The figure shows three views and two pictorial views of one solid part (mm, origin at its lowest corner). Answer the questions. A direction names the side the tool comes from. Coordinates: 2 decimals unless noted, no trailing zeros. Order: outer loops, then holes, each group sorted by start corner. A loop starts at its lowest first (then second) coordinate and runs counter-clockwise, first axis right, second up.
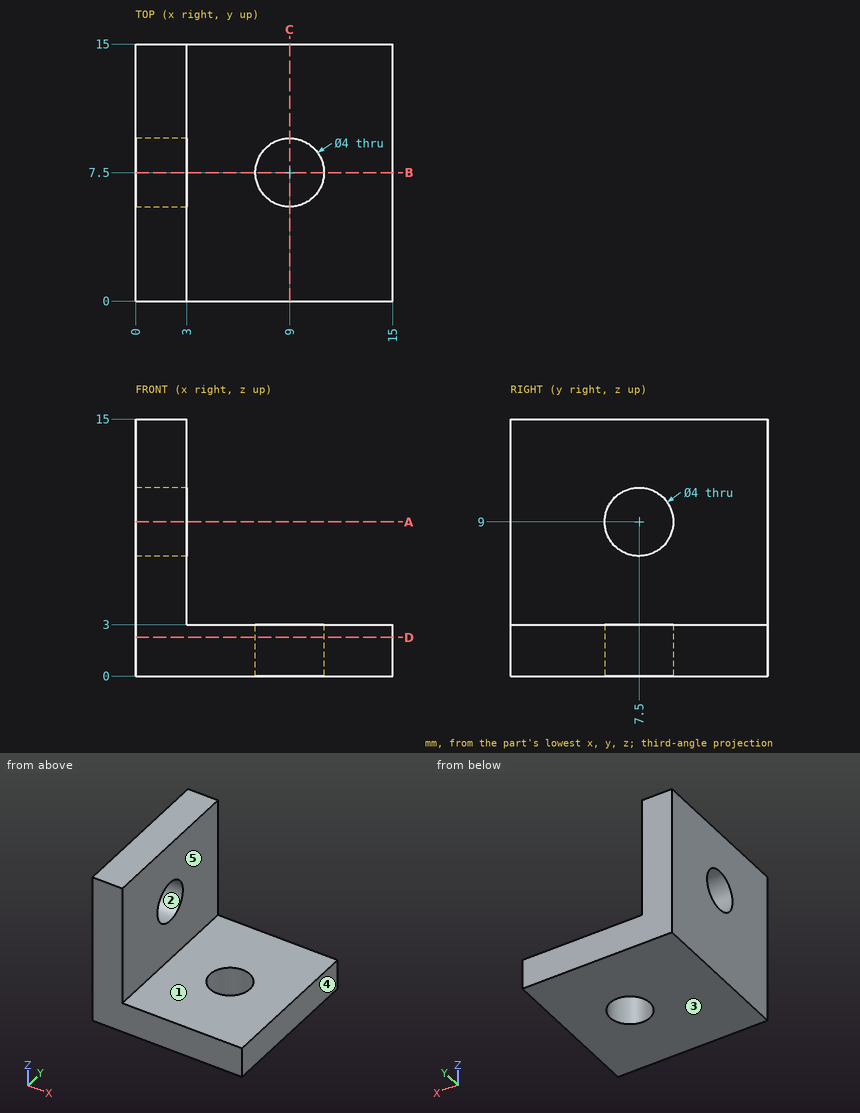
Q1. This flat-tipped pin is pushed along its axis until it touches: P1, Ø1, axis at x = 9.5, y = 7, coming from the +Z side. Where does it stop, or does it pass through?
Q2. The part is cut by section D-D, the plane z = 2.25. Determine the outline of the cut face in (x, y).
Q3. The part is cut by section A-A, the plane z = 9. Determine the outline of the cut face in (x, y), then the cut area to 3 significant figures.
Q4. Determine the mould class of the marked faces 1, 2 and 3 for opening direction Z: +Z half, -Z half, draft (parallel to the pull), parting line (faces both ways), or undercut.
Q5. Straight lines are drawn through the part: L1, parallel to Z at x = 0.75, y = 7.5; L2, parallel to Y at x = 9, z = 0.95; L3, parallel to Z at x = 6.5, y = 6.5. For each, find the intervals that lie inside material, in ascending order.
Q6. Which of the six approach directions +Z, -Z, +X, -X, +Y, -Y give full straight-line access (tool end or side, diameter ignored) to the marked faces 4 and 5?
Q7. The part is cut by section C-C, the plane x = 9. Determine the outline of the cut face in (y, z).
Q8. The part is cut by section B-B, the plane y = 7.5. Determine the outline of the cut face in (x, z), then the cut area to 3 significant figures.
Computed values:
1. P1: passes through
2. outline: (0, 0) - (15, 0) - (15, 15) - (0, 15) - close; hole circle Ø4 at (9, 7.5)
3. outline: (0, 0) - (3, 0) - (3, 5.5) - (0, 5.5) - close; (0, 9.5) - (3, 9.5) - (3, 15) - (0, 15) - close
3. area: 33.0 mm2
4. face 1: +Z half
4. face 2: undercut
4. face 3: -Z half
5. L1: z = 0 to 7, 11 to 15
5. L2: y = 0 to 5.5, 9.5 to 15
5. L3: z = 0 to 3
6. face 4: +Z, -Z, +X, +Y, -Y
6. face 5: +Z, +X, +Y, -Y
7. outline: (0, 0) - (5.5, 0) - (5.5, 3) - (0, 3) - close; (9.5, 0) - (15, 0) - (15, 3) - (9.5, 3) - close
8. outline: (0, 0) - (7, 0) - (7, 3) - (3, 3) - (3, 7) - (0, 7) - close; (0, 11) - (3, 11) - (3, 15) - (0, 15) - close; (11, 0) - (15, 0) - (15, 3) - (11, 3) - close
8. area: 57.0 mm2
